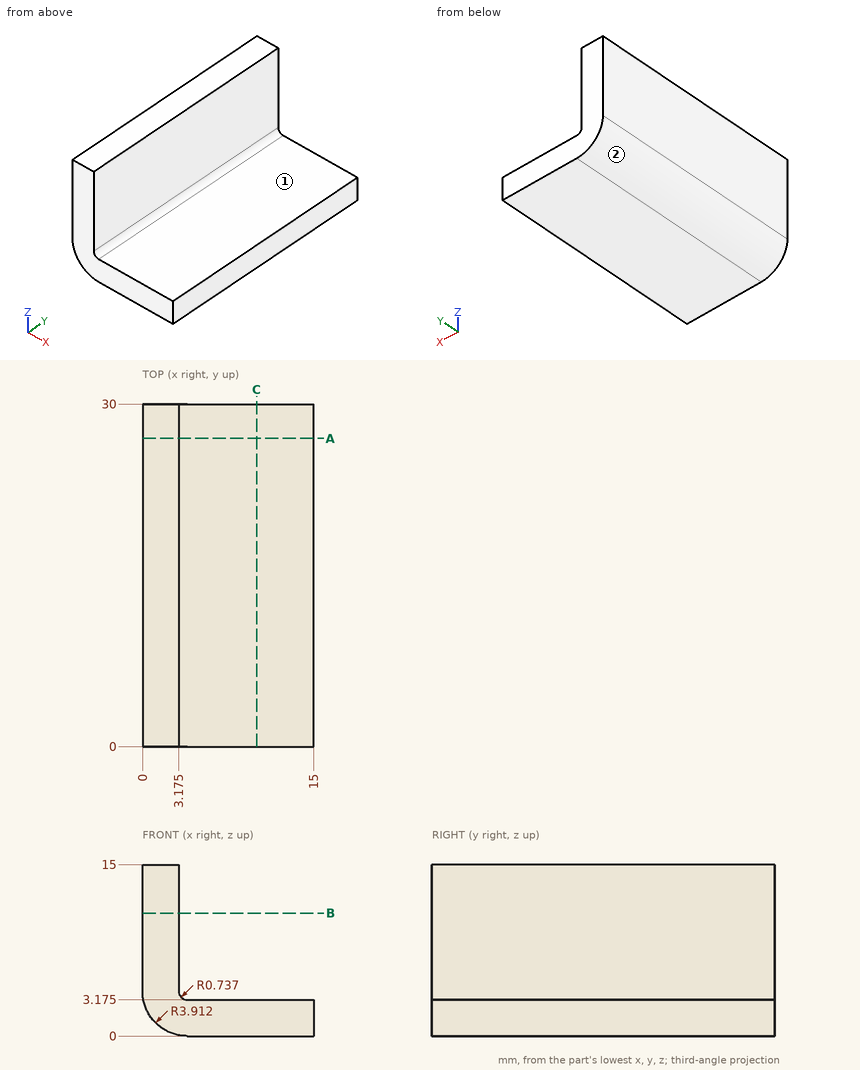
Study the drawing (mm; zero at the part's minimum x, y, z) and answer. A direction names the side the tool comes from. Give positions to 0.01 mm unless a question says otherwise; leave off trailing zeros. Write each loop counter-clockwise with the first axis right and the second up, starting at its lowest first coordinate (ties: lowest second). Pieces come first, ordered by that corner, then holes. Notation, with made-up numbers: M 12,-4.75 L 24,-4.75 A35 ccw 24,32.25 Z; hole C 25,3.25 d4. An arc over 180 degrees is marked long. Put each result on its own line as item: value. Start each with the question number.
1. The part is cut by section A-A, the plane y = 27. Give the vertices of the cut face in (x, z) (1 decimal).
2. Which of the six approach directions +Z, -Z, +X, -X, +Y, -Y give full straight-line access (tool end or side, diameter ignored) to the marked faces 1 and 2?
3. Consider line 1 along Z through (x, y) = (13, 26.25) (1 decimal); line 2 along Z through (x, y) = (2.5, 5.25) (1 decimal). Determine where each line is inside the solid, lowest interval first.
4. Each of these flat-tipped pins is pushed along its axis until it touches: pin 1 Ø9 at (y, z) = (10.5, 7.5) entering from +X; pin 2 Ø1.5 at (x, z) = (8, 4.5) entering from +Y; pin 3 Ø3 at (y, z) = (8, 8.5) entering from +X (3 decimals); pin 4 Ø5 at (x, y) = (7.5, 25) entering from +Z (3 decimals). Where does it stop, or does it pass through?
5. The part is cut by section C-C, the plane x = 10. Give the vertices of the cut face in (y, z) (1 decimal).
6. The part is cut by section B-B, the plane z = 10.75. Give the vertices of the cut face in (x, y) (1 decimal).
Final values:
1. outline: M 0,3.9 A3.9 ccw 3.9,0 L 15,0 L 15,3.2 L 3.9,3.2 A0.7 cw 3.2,3.9 L 3.2,15 L 0,15 Z
2. face 1: +Z, +X, +Y, -Y
2. face 2: -Z, -X, +Y, -Y
3. line 1: z = 0 to 3.2
3. line 2: z = 0.3 to 15
4. pin 1: stops at x = 15
4. pin 2: passes through
4. pin 3: stops at x = 3.175
4. pin 4: stops at z = 3.175
5. outline: M 0,0 L 30,0 L 30,3.2 L 0,3.2 Z
6. outline: M 0,0 L 3.2,0 L 3.2,30 L 0,30 Z
